Verification items for the finished model (mm, model axes). A direction names the side the tool comes from. Coordinates: 2 decimals unless noted, no trailing zeros. Order: outer loops, then holes, each group sorted by start corner. A loop starts at its lowest first (then second) coordinate and runs counter-clockwise, first axis right, second up. Notation, with made-up numbers: M 70.5,23.5 L 83.5,23.5 A10 ccw 83.5,30.5 Z; hole C 9,-5 d9. An arc over 180 degrees is marked long. Use one line per item in the form item = value. Start each with the question number.
Autodesk Inventor part; units mm, degrees
ref_plane "YZ Plane" through (0, 0, 0) normal (1, 0, 0) x (0, 1, 0)
ref_plane "XZ Plane" through (0, 0, 0) normal (0, 1, 0) x (-1, 0, 0)
ref_plane "XY Plane" through (0, 0, 0) normal (0, 0, 1) x (1, 0, 0)
sketch "Sketch1" plane through (0, 0, 0) normal (0, 0, 1) x (1, 0, 0)
  line L0 (0, 0) -> (80, 0)
  line L1 (80, 0) -> (80, 60)
  line L2 (80, 60) -> (0, 60)
  line L3 (0, 60) -> (0, 0)
  dimension "d0" = 80
  dimension "d1" = 60
extrude "Extrusion1" add sketch "Sketch1" along normal blind 138
shell "Shell1" thickness 10 removed faces 3 at (53.3333, 60, 46) at (26.6667, 40, 138) at (26.6667, 40, 0)
fillet "Fillet1" radius 10 2 edges at (10, 10, 69) (70, 10, 69)
fillet "Fillet2" radius 20 1 edges at (80, 0, 69)
fillet "Fillet3" radius 20 1 edges at (0, 0, 69)
sketch "Sketch2" plane through (80, 60, 138) normal (1, 0, 0) x (0, 0, -1)
  point P0 (138, -60)
fillet "Fillet4" radius 15 1 edges at (75, 60, 0)
fillet "Fillet5" radius 15 1 edges at (75, 60, 138)
fillet "Fillet6" radius 5 1 edges at (5, 60, 138)
fillet "Fillet7" radius 5 1 edges at (5, 60, 0)
sketch "Sketch5" plane through (20, 10, 0) normal (0, 1, 0) x (1, 0, 0)
  line L0 (40, -138) -> (0, -138)
  line L1 (0, 0) -> (40, 0)
  circle A0 centre (20, -130) radius 1.5
  circle A1 centre (20, -10) radius 1.5
  point P0 (-20, 0)
  dimension "d13" = 3
  dimension "d15" = 3
extrude "Extrusion2" cut sketch "Sketch5" against normal through all
thread "Thread1"
thread "Thread2"
sketch "Sketch6" plane through (20, 10, 0) normal (0, 1, 0) x (1, 0, 0)
  point P0 (-20, 0)
properties part number "BREAD"
1. Cross-section at B-B on y = 25. Enter the section's corners in (x, z).
2. Release check for a two-part mould opening along X. For faces 1 (the flat face through (10, 40, 68)), 2 (the flat face through (0, 40, 68)), 3 (the flat face through (75, 60, 68)) record: pulls with the +X half, pulls with the -X half, needs draft (parallel to the pull), parting line crosses it, or undercut.
3. Cross-section at A-A on x = 40. Enter the section's corners in (y, z), and give its area (3 significant figures).
4. Cross-section at C-C on z = 103.5. Enter the section's corners in (x, y).
5. Tool access check on faces 4 (the cylindrical face through (5.703, 6.014, 69.966)), 5 (the cylindrical face through (12.85, 13.01, 69.97)), 6 (the cylindrical face through (74.93, 55.72, 4.51)), 7 (the flat face through (40, 9, 138)), 8 (the cylindrical face through (74.93, 55.49, 133.72)). Record the directions out of +Z, -Z, +X, -X, +Y, -Y that give a thin tool (end or side, any length) a straight path to the whole face; none if there is none.
6. Depth check by flat-ended pin: P1, Ø4, axis at x = 55, z = 33.5, coming from the +Y side; P2, Ø1.5, axis at x = 62, z = 58, coming from the -Y side; P3, Ø8, axis at y = 15.5, z = 24, coming from the +X side. Enter the tip coordinate at first touch or a pass-through.
7. Material ranges on line 1 along Z through (x, y) = (40, 7.5); line 2 along X through (y, z) = (27, 40); line 3 along Z through (x, y) = (41, 2), recorded low to high.
8. Cross-section at D-D on z = 130. Enter the section's corners in (x, y).
Final values:
q1.outline = M 0,0 L 10,0 L 10,138 L 0,138 Z; M 70,0 L 80,0 L 80,138 L 70,138 Z
q2.face_1 = undercut
q2.face_2 = pulls with the -X half
q2.face_3 = needs draft
q3.outline = M 0,0 L 10,0 L 10,8.5 L 0,8.5 Z; M 0,11.5 L 10,11.5 L 10,128.5 L 0,128.5 Z; M 0,131.5 L 10,131.5 L 10,138 L 0,138 Z
q3.area = 1,320 mm2
q4.outline = M 0,20 A20 ccw 20,0 L 60,0 A20 ccw 80,20 L 80,60 L 70,60 L 70,20 A10 cw 60,10 L 20,10 A10 cw 10,20 L 10,60 L 0,60 Z
q5.face_4 = +Z, -Z, -X, -Y
q5.face_5 = +Z, -Z, +Y
q5.face_6 = -Z, +X, +Y
q5.face_7 = +Z, +X, -X, +Y, -Y
q5.face_8 = +Z, +X, +Y
q6.P1 = 10
q6.P2 = 0.04
q6.P3 = 79.99
q7.line_1 = 0 to 8.5, 11.5 to 128.5, 131.5 to 138
q7.line_2 = 0 to 10, 70 to 80
q7.line_3 = 0 to 8.88, 11.12 to 128.88, 131.12 to 138
q8.outline = M 0,20 A20 ccw 20,0 L 38.5,0 L 38.5,10 L 20,10 A10 cw 10,20 L 10,60 L 0,60 Z; M 41.5,0 L 60,0 A20 ccw 80,20 L 80,58.27 L 70,58.27 L 70,20 A10 cw 60,10 L 41.5,10 Z
